```python
from build123d import *

# Parameters (mm, degrees)
SKETCH1_R           = 2
BOSS_EXTRUDE1_DEPTH = 5
BOSS_EXTRUDE2_DEPTH = 10
SKETCH3_R           = 4
CUT_EXTRUDE1_DEPTH  = 16
BOSS_EXTRUDE3_DEPTH = 16
SKETCH5_R           = 4
CUT_EXTRUDE2_DEPTH  = 23
SKETCH7_W           = 35
SKETCH7_H           = 10
BOSS_EXTRUDE4_DEPTH = 10
BOSS_EXTRUDE5_DEPTH = 35
SKETCH10_W          = 35
SKETCH10_H          = 10
BOSS_EXTRUDE6_DEPTH = 10
BOSS_EXTRUDE7_DEPTH = 35


with BuildPart() as part:
    # Sketch1 → Boss-Extrude1 (new body)
    with BuildSketch(Plane(origin=(0, 0, 0), x_dir=(1, 0, 0), z_dir=(0, 1, 0))):
        with BuildLine():
            Line((-35, 20), (35, 20))
            ThreePointArc((35, 20), (38.535533906, 18.535533906), (40, 15))
            Line((40, 15), (40, -15))
            ThreePointArc((40, -15), (38.535533906, -18.535533906), (35, -20))
            Line((35, -20), (-35, -20))
            ThreePointArc((-35, -20), (-38.535533906, -18.535533906), (-40, -15))
            Line((-40, -15), (-40, 15))
            ThreePointArc((-40, 15), (-38.535533906, 18.535533906), (-35, 20))
        make_face()
        with Locations((-35, 15)):
            Circle(SKETCH1_R, mode=Mode.SUBTRACT)
        with Locations((-35, -15)):
            Circle(SKETCH1_R, mode=Mode.SUBTRACT)
        with Locations((35, 15)):
            Circle(SKETCH1_R, mode=Mode.SUBTRACT)
        with Locations((35, -15)):
            Circle(SKETCH1_R, mode=Mode.SUBTRACT)
    extrude(amount=BOSS_EXTRUDE1_DEPTH)

    # Sketch2 → Boss-Extrude2 (add)
    with BuildSketch(Plane(origin=(40, 0, 0), x_dir=(0, 0, -1), z_dir=(1, 0, 0))):
        with BuildLine():
            ThreePointArc((10, 15), (0, 25), (-10, 15))
            Line((-10, 15), (-10, 0))
            Line((-10, 0), (10, 0))
            Line((10, 0), (10, 15))
        make_face()
    extrude(amount=-BOSS_EXTRUDE2_DEPTH)

    # Sketch3 → Cut-Extrude1 (cut)
    with BuildSketch(Plane(origin=(40, 0, 0), x_dir=(0, 0, -1), z_dir=(1, 0, 0))):
        with Locations((0, 15)):
            Circle(SKETCH3_R)
    extrude(amount=-CUT_EXTRUDE1_DEPTH, mode=Mode.SUBTRACT)

    # Sketch4 → Boss-Extrude3 (add)
    with BuildSketch(Plane.ZY.offset(40)):
        with BuildLine():
            Line((0, 0), (-10, 0))
            Line((-10, 0), (-10, 15))
            ThreePointArc((-10, 15), (0, 25), (10, 15))
            Line((10, 15), (10, 0))
            Line((10, 0), (0, 0))
        make_face()
    extrude(amount=-BOSS_EXTRUDE3_DEPTH)

    # Sketch5 → Cut-Extrude2 (cut)
    with BuildSketch(Plane.ZY.offset(40)):
        with Locations((0, 15)):
            Circle(SKETCH5_R)
    extrude(amount=-CUT_EXTRUDE2_DEPTH, mode=Mode.SUBTRACT)

    # Sketch7 → Boss-Extrude4 (add)
    with BuildSketch(Plane(origin=(0, 5, 0), x_dir=(1, 0, 0), z_dir=(0, 1, 0))):
        with Locations((0, 15)):
            Rectangle(SKETCH7_W, SKETCH7_H)
    extrude(amount=BOSS_EXTRUDE4_DEPTH)

    # Sketch8 → Boss-Extrude5 (add)
    with BuildSketch(Plane.ZY.offset(17.5)):
        with BuildLine():
            Line((-20, 15), (-10, 15))
            ThreePointArc((-10, 15), (-15, 20), (-20, 15))
        make_face()
    extrude(amount=-BOSS_EXTRUDE5_DEPTH)

    # Sketch10 → Boss-Extrude6 (add)
    with BuildSketch(Plane(origin=(0, 5, 0), x_dir=(1, 0, 0), z_dir=(0, 1, 0))):
        with Locations((0, -15)):
            Rectangle(SKETCH10_W, SKETCH10_H)
    extrude(amount=BOSS_EXTRUDE6_DEPTH)

    # Sketch11 → Boss-Extrude7 (add)
    with BuildSketch(Plane(origin=(17.5, 0, 0), x_dir=(0, 0, -1), z_dir=(1, 0, 0))):
        with BuildLine():
            Line((-20, 15), (-10, 15))
            ThreePointArc((-10, 15), (-15, 20), (-20, 15))
        make_face()
    extrude(amount=-BOSS_EXTRUDE7_DEPTH)


solid = part.part
```
Geometry check sheet. Reference: the model listing, model coordinates, mm. A direction names the side the tool comes from. Round coordinates to 2 decimals unless told otherwise and drop trailing zeros. Loops run counter-clockwise (first coordinate to the right, second up) from the corner with the lowest first, then second, coordinate; pieces in that order, holes last. Notation, with made-up numbers: (-12.5, -26.5) - (14.5, -26.5) arc R24 cw to (14.5, 0.5) - close; hole circle Ø7 at (18.25, 30.25). An arc over 180 degrees is marked (long way). Write item = value, one per line. Start each with the question number.
1. Depth check by flat-ended pin: pin 1 (3 mm diameter, centred on x = -35, y = 8.5, fed in from +Z); pin 2 (5 mm diameter, centred on y = 21.5, z = 13.5, fed in from +X); pin 3 (6 mm diameter, centred on x = -25, y = 14, fed in from -Z). Enter the tip coordinate at first touch or a pass-through.
2. Section check A-A on z = 0. Enter the section's corners in (x, y), then the cut area to 3 significant figures.
3. Thickness scan on line 1 (X direction, y = 1.8, z = 15); line 2 (Z direction, x = -35, y = 3.6); line 3 (Z direction, x = -9, y = 7). Record the ranges inside material, lowest first.
4. Mould release check, pull along Z, two halves, no side actions. Record for faces 6 (the face through (0, 20, 15)), 7 (the face through (30, 10.7, 0.1)), 8 (the face through (36.908, 2.465, -15.601)), 9 (the face through (-32, 25, 0)): released by +Z, released by -Z, zero draft, split by the parting line, or undercut.
5. Section check B-B on x = -32. Enter the section's corners in (y, z).
6. Set-up check for faces 1 (the face through (-32, 10, 10)), 2 (the face through (35.07, 18.966, 0.521)), 3 (the face through (-32, 10, -10)), 4 (the face through (-17.5, 13, -15)), 5 (the face through (0, 10, 10)): record each of +Z, -Z, +X, -X, +Y, -Y from which the full face is reachable in a straight line by a thin tool's end or side.
7. Section check D-D on y = 22.75. Enter the section's corners in (x, z).
8. Section check C-C on y = 6. Enter the section's corners in (x, z).
Working result:
q1.pin_1 = 10
q1.pin_2 = 17.5
q1.pin_3 = -10
q2.outline = (-40, 0) - (40, 0) - (40, 11) - (30, 11) - (30, 5) - (-24, 5) - (-24, 11) - (-40, 11) - close; (-40, 19) - (-24, 19) - (-24, 25) - (-40, 25) - close; (30, 19) - (40, 19) - (40, 25) - (30, 25) - close
q2.area = 712 mm^2
q3.line_1 = -40 to -37, -33 to 33, 37 to 40
q3.line_2 = -20 to -17, -13 to 13, 17 to 20
q3.line_3 = -20 to -10, 10 to 20
q4.face_6 = undercut
q4.face_7 = zero draft
q4.face_8 = undercut
q4.face_9 = split by the parting line
q5.outline = (0, -20) - (5, -20) - (5, -10) - (15, -10) arc R10 ccw to (15, 10) - (5, 10) - (5, 20) - (0, 20) - close; hole circle Ø8 at (15, 0)
q6.face_1 = +Z, -X, +Y
q6.face_2 = +X, -X
q6.face_3 = -Z, -X, +Y
q6.face_4 = +Z, -Z, -X, +Y
q6.face_5 = +Y
q7.outline = (-40, -6.32) - (-24, -6.32) - (-24, 6.32) - (-40, 6.32) - close; (30, -6.32) - (40, -6.32) - (40, 6.32) - (30, 6.32) - close
q8.outline = (-40, -10) - (-24, -10) - (-24, 10) - (-40, 10) - close; (-17.5, -20) - (17.5, -20) - (17.5, -10) - (-17.5, -10) - close; (-17.5, 10) - (17.5, 10) - (17.5, 20) - (-17.5, 20) - close; (30, -10) - (40, -10) - (40, 10) - (30, 10) - close
